Print and shaded views of the part. All mm, measured from the part's lowest x, y and z. Coordinates: 2 decimals unless noted, no trailing zeros. Loops run counter-clockwise (first coordinate to the right, second up) from the corner with the lowest first, then second, coordinate; pieces in that order, holes last. Notation, with made-up numbers: (57.25, 50) -> (68.25, 50) arc R22 cw to (68.25, 74) -> close; hole circle Ø2 at (76.5, 32). An arc over 180 degrees is marked (long way). One line per item, written item: value. Start each with the question number.
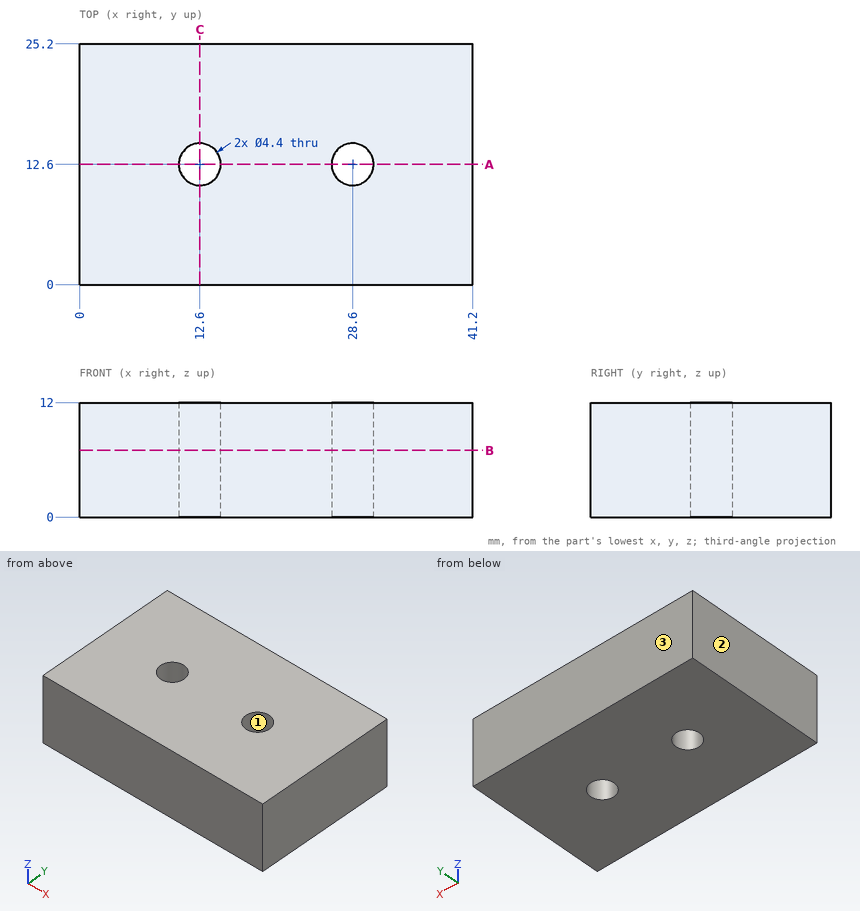
1) Slice it at C-C (x = 12.6). Give the cut face in (y, z), then the cut area to 3 significant figures.
2) Slice it at A-A (y = 12.6). Give the cut face in (x, z), then the cut area to 3 significant figures.
3) Probe line 1 (X direction, y = 12.5, z = 5.75); line 2 (X direction, y = 13.75, z = 9.25); line 3 (Y direction, x = 28.6, z = 6.5). List the from-to ranges inside material, lowest first. Write a range as from..to.
4) Pin check, flat tip, straight feed: pin 1 Ø10 at (x, y) = (17, 11.5) entering from -Z. Stop position of the tip, or through.
5) Slice it at B-B (z = 7). Give the cut face in (x, y), then the cut area to 3 significant figures.
6) Pull direction Y, two halves, no side cores. Call the marked faces 1, 2 and 3: +Y half, -Y half, draft (parallel to the pull), parting line (faces both ways), or undercut.
Check sheet entries:
1. outline: (0, 0) -> (10.4, 0) -> (10.4, 12) -> (0, 12) -> close; (14.8, 0) -> (25.2, 0) -> (25.2, 12) -> (14.8, 12) -> close
1. area: 250 mm^2
2. outline: (0, 0) -> (10.4, 0) -> (10.4, 12) -> (0, 12) -> close; (14.8, 0) -> (26.4, 0) -> (26.4, 12) -> (14.8, 12) -> close; (30.8, 0) -> (41.2, 0) -> (41.2, 12) -> (30.8, 12) -> close
2. area: 389 mm^2
3. line 1: x = 0..10.4, 14.8..26.4, 30.8..41.2
3. line 2: x = 0..10.72, 14.48..26.72, 30.48..41.2
3. line 3: y = 0..10.4, 14.8..25.2
4. pin 1: stops at z = 0
5. outline: (0, 0) -> (41.2, 0) -> (41.2, 25.2) -> (0, 25.2) -> close; hole circle Ø4.4 at (12.6, 12.6); hole circle Ø4.4 at (28.6, 12.6)
5. area: 1,010 mm^2
6. face 1: undercut
6. face 2: draft
6. face 3: +Y half
